Work out the finished part from the listing and answer in its coordinate system (mm). Give positions to 0.01 mm unless a question says otherwise; leave off trailing zeros. Order: outer loops, then holes, each group sorted by start corner. A loop starts at its lowest first (then second) coordinate and runs counter-clockwise, first axis right, second up.
```python
from build123d import *

# Parameters (mm, degrees)
BOX048_W          = 10
BOX048_H          = 10
BOX048_DEPTH      = 6.5
CYLINDER028_R     = 4.4
CYLINDER028_DEPTH = 16


with BuildPart() as cube010:
    # Box048 → Box048 (new body)
    with BuildSketch(Plane(origin=(22.5, -99.5, -31), x_dir=(1, 0, 0), z_dir=(0, 0, 1))):
        with Locations((5, 5)):
            Rectangle(BOX048_W, BOX048_H)
    extrude(amount=BOX048_DEPTH)


with BuildPart() as cone:
    # Cone → Cone (revolve)
    with BuildSketch(Plane(origin=(27.5, -94.5, 71), x_dir=(1, 0, 0), z_dir=(0, -1, 0))):
        Polygon((0, 0), (1.75, 0), (3.5, 16), (0, 16), align=None)
    revolve(axis=Axis((27.5, -94.5, 71), (0, 0, 1)))


with BuildPart() as cut007:
    # Cylinder028 → Cylinder028 (new body)
    with BuildSketch(Plane(origin=(27.5, -94.5, 71), x_dir=(1, 0, 0), z_dir=(0, 0, 1))):
        Circle(CYLINDER028_R)
    extrude(amount=CYLINDER028_DEPTH)

    # Cut006: cut Cone
    add(cone.part, mode=Mode.SUBTRACT)


with BuildPart() as cut007_1:
    # Cut006 placement: moved
    add(cut007.part.moved(Location((0, 0, -111.5))))

    # Cut007: cut Cube010
    add(cube010.part, mode=Mode.SUBTRACT)


solid = cut007_1.part
```
1. The part is cut by section D-D (x = 31.75). Write down the section's boundary in (y, z), then the cut area to 3 significant figures.
Findings below:
outline: (-95.64, -40.5) - (-93.36, -40.5) - (-93.36, -31) - (-95.64, -31) - close
area: 21.6 mm2
2. Straight lines are drawn through the part: probe 1 along Y at (x, z) = (27.25, -34); probe 2 along Y at (x, z) = (27.75, -36.75); probe 3 along X at (y, z) = (-96.5, -34.5). For each, find the intervals that lie inside material, in ascending order.
Findings below:
probe 1: y = -98.89 to -96.95, -92.05 to -90.11
probe 2: y = -98.89 to -96.65, -92.35 to -90.11
probe 3: x = 23.58 to 26.16, 28.84 to 31.42
3. Given P1, Ø4, axis at x = 30, z = -36, coming from the -Y side; P2, Ø1.5, axis at x = 25, z = -34.5, coming from the +Y side; P3, Ø5, axis at x = 27, y = -96, coming from the +Z side, each flat-ended and moving along its own axis, determine where each tip first touches the part or whether it passes through.
Findings below:
P1: stops at y = -98.87
P2: stops at y = -90.46
P3: stops at z = -31
4. The part is cut by section B-B (y = -94.5). Write down the section's boundary in (x, z), then the cut area to 3 significant figures.
Findings below:
outline: (23.1, -40.5) - (25.75, -40.5) - (24.71, -31) - (23.1, -31) - close; (29.25, -40.5) - (31.9, -40.5) - (31.9, -31) - (30.29, -31) - close
area: 40.5 mm2
5. The part is cut by section A-A (x = 27.5). Write down the section's boundary in (y, z).
Findings below:
outline: (-98.9, -40.5) - (-96.25, -40.5) - (-97.29, -31) - (-98.9, -31) - close; (-92.75, -40.5) - (-90.1, -40.5) - (-90.1, -31) - (-91.71, -31) - close
6. The part is cut by section C-C (z = -38.5). Write down the section's boundary in (x, y).
Findings below:
outline: circle Ø8.8 at (27.5, -94.5); hole circle Ø3.94 at (27.5, -94.5)
